```python
from build123d import *

# Parameters (mm, degrees)
F0_W      = 325.4248
F0_H      = 261.9248
F1_DEPTH  = 242.8748
F2_W      = 317.5
F2_H      = 254
F3_DEPTH  = 234.95
F5_DEPTH  = 698.5
F7_W      = 127
F7_H      = 254
F8_DEPTH  = 3.9624
F10_W     = 325.4248
F10_H     = 261.9248
F11_DEPTH = 3.9624
F13_DEPTH = 338.328


with BuildPart() as f1:
    # F0 (on Top) → F1 (new body)
    with BuildSketch(Plane.XY):
        Rectangle(F0_W, F0_H)
    extrude(amount=F1_DEPTH)

    # F2 (on face) → F3 (cut)
    with BuildSketch(Plane.XY.offset(242.8748)):
        Rectangle(F2_W, F2_H)
    extrude(amount=-F3_DEPTH, mode=Mode.SUBTRACT)

    # F4 (on face) → F5 (cut)
    with BuildSketch(Plane.YZ.offset(162.7124)):
        Polygon((127, 3.9624), (0.79375, 3.9624), (-0.79375, 3.9624), (-127, 3.9624), (-127, 3.5814), (-0.79375, 3.5814), (-0.79375, -3.9624), (0.79375, -3.9624), (0.79375, 3.5814), (127, 3.5814), align=None)
    extrude(amount=-F5_DEPTH, mode=Mode.SUBTRACT)

    # F7 (on offset) → F8 (join)
    with BuildSketch(Plane.XY.offset(3.9878)):
        with Locations((95.25, 0)):
            Rectangle(F7_W, F7_H)
        with Locations((-95.25, 0)):
            Rectangle(F7_W, F7_H)
    extrude(amount=F8_DEPTH)

    # F10 (on face) → F11 (join)
    with BuildSketch(Plane.XY.offset(242.8748)):
        Rectangle(F10_W, F10_H)
    extrude(amount=-F11_DEPTH)

    # F12 (on face) → F13 (cut)
    with BuildSketch(Plane.YZ.offset(162.7124)):
        Polygon((0, 242.8748), (-0.79375, 242.8748), (-0.79375, 239.2934), (-127, 239.2934), (-127, 238.9124), (0, 238.9124), align=None)
        Polygon((0.79375, 242.8748), (0, 242.8748), (0, 238.9124), (127, 238.9124), (127, 239.2934), (0.79375, 239.2934), align=None)
    extrude(amount=-F13_DEPTH, mode=Mode.SUBTRACT)


solid = f1.part
```
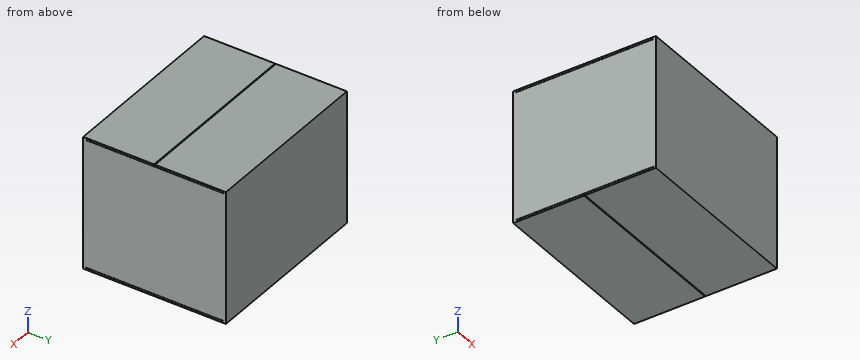
CAD build for the part. Positions are in the model's coordinates, mm. Round coordinates to 2 decimals unless told otherwise and drop trailing zeros. Write each loop counter-clockwise with the first axis right and the second up, starting at its lowest first coordinate (ties: lowest second). Pieces come first, ordered by that corner, then holes. Notation, with made-up numbers: M -36.5,81 L -9.5,81 A21 cw -9.5,104 Z; hole C -38,4.5 d5. An arc over 180 degrees is marked long. One line per question, with ' | ' between items.
1. Cut at B-B on x = 118.5. Write the cut outline in (y, z), and give its area (3 significant figures).
Working result:
outline: M -130.96,0 L -0.79,0 L -0.79,3.58 L -127,3.58 L -127,3.96 L 127,3.96 L 127,3.58 L 0.79,3.58 L 0.79,0 L 130.96,0 L 130.96,242.87 L 0.79,242.87 L 0.79,239.29 L 127,239.29 L 127,7.95 L -127,7.95 L -127,239.29 L -0.79,239.29 L -0.79,242.87 L -130.96,242.87 Z | area: 4,750 mm2
2. Probe L1, parallel to Z at x = 146, y = -2; L2, parallel to Z at x = 27, y = -68; L3, parallel to X at y = 81, z = 215.5. List the from-to ranges inside material, lowest first. Write a range as from..to.
Working result:
L1: 0..3.58, 3.96..7.95, 239.29..242.87 | L2: 0..3.58, 3.96..7.92, 239.29..242.87 | L3: -162.71..-158.75, 158.75..162.71
3. Cut at C-C on z = 223. Write the cut outline in (x, y).
Working result:
outline: M -162.71,-130.96 L 162.71,-130.96 L 162.71,130.96 L -162.71,130.96 Z; hole M -158.75,-127 L 158.75,-127 L 158.75,127 L -158.75,127 Z
4. Cut at D-D on x = -21. Write the cut outline in (y, z), and give its area (3 significant figures).
Working result:
outline: M -130.96,0 L -0.79,0 L -0.79,3.58 L -127,3.58 L -127,3.96 L 127,3.96 L 127,3.58 L 0.79,3.58 L 0.79,0 L 130.96,0 L 130.96,242.87 L 0.79,242.87 L 0.79,239.29 L 127,239.29 L 127,7.92 L -127,7.92 L -127,239.29 L -0.79,239.29 L -0.79,242.87 L -130.96,242.87 Z | area: 4,740 mm2
5. Cut at A-A on y = 81. Count the separate pieces of the cut face and the enclosed holes in it, and give its area (3 significant figures).
Working result:
separate pieces: 3 | enclosed holes: 0 | area: 5,460 mm2
